```python
from build123d import *

# Parameters (mm, degrees)
CYLINDER001_R     = 1.5
CYLINDER001_DEPTH = 14
CYLINDER_R        = 1.5
CYLINDER_DEPTH    = 14
BOX003_W          = 3
BOX003_H          = 6.8
BOX003_DEPTH      = 6
BOX002_W          = 3
BOX002_H          = 6.8
BOX002_DEPTH      = 6
BOX001_W          = 3
BOX001_H          = 65
BOX001_DEPTH      = 6


with BuildPart() as cylinder001:
    # Cylinder001 → Cylinder001 (new body)
    with BuildSketch(Plane(origin=(-13, 30.6, 0), x_dir=(0, 0, -1), z_dir=(1, 0, 0))):
        Circle(CYLINDER001_R)
    extrude(amount=CYLINDER001_DEPTH)


with BuildPart() as cylinder:
    # Cylinder → Cylinder (new body)
    with BuildSketch(Plane(origin=(-13, -27.6, 0), x_dir=(0, 0, -1), z_dir=(1, 0, 0))):
        Circle(CYLINDER_R)
    extrude(amount=CYLINDER_DEPTH)


with BuildPart() as cube003:
    # Box003 → Box003 (new body)
    with BuildSketch(Plane(origin=(-6, -31, -3), x_dir=(1, 0, 0), z_dir=(0, 0, 1))):
        with Locations((1.5, 3.4)):
            Rectangle(BOX003_W, BOX003_H)
    extrude(amount=BOX003_DEPTH)


with BuildPart() as cube002:
    # Box002 → Box002 (new body)
    with BuildSketch(Plane(origin=(-6, 27.2, -3), x_dir=(1, 0, 0), z_dir=(0, 0, 1))):
        with Locations((1.5, 3.4)):
            Rectangle(BOX002_W, BOX002_H)
    extrude(amount=BOX002_DEPTH)


with BuildPart() as cut002:
    # Box001 → Box001 (new body)
    with BuildSketch(Plane(origin=(-3, -31, -3), x_dir=(1, 0, 0), z_dir=(0, 0, 1))):
        with Locations((1.5, 32.5)):
            Rectangle(BOX001_W, BOX001_H)
    extrude(amount=BOX001_DEPTH)

    # Fusion: union Cube003, Cube002
    add(cube003.part)
    add(cube002.part)

    # Cut001: cut Cylinder
    add(cylinder.part, mode=Mode.SUBTRACT)

    # Cut002: cut Cylinder001
    add(cylinder001.part, mode=Mode.SUBTRACT)


solid = cut002.part
```
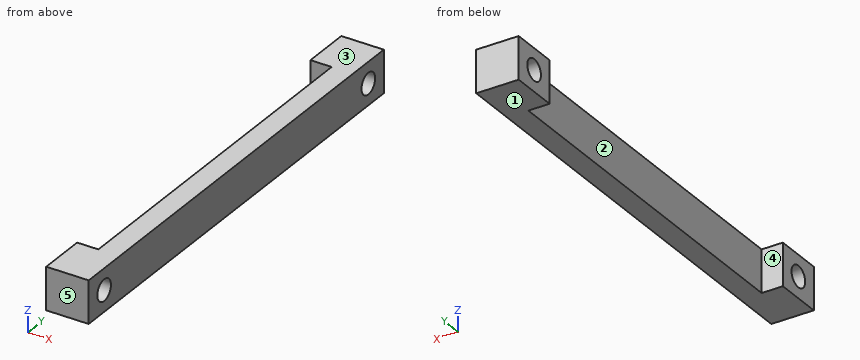
Geometry check sheet. Reference: the model listing, model coordinates, mm. Face numbers are marked on the shaded views. A direction names the side the tool comes from. Coordinates: 2 decimals unless noted, no trailing zeros. Order: outer loops, then holes, each group sorted by start corner. A loop starts at its lowest first (then second) coordinate and runs counter-clockwise, first axis right, second up. Notation, with made-up numbers: (65, 33.25) - (96, 33.25) arc R11 cw to (96, 54.25) - close; hole circle Ø11 at (-6, 3.5). An arc over 180 degrees is marked (long way). Answer in a Markdown table with one row per item. Add a question column.
1. Section check B-B (z = 0). Enter the section's corners in (x, y).
2. Section check C-C (y = -27.6). Enter the section's corners in (x, z), plus the area to 3 significant figures.
3. Section check A-A (x = -4.45). Enter the section's corners in (y, z).
4. Access from +Z, -Z, +X, -X, +Y, -Y to the whole of each face (thin tool, end or side, straight path). Record for the marked faces 1 and 2.
5. Material ranges on L1, parallel to Y at x = -2.5, z = 0; L2, parallel to Y at x = -3.8, z = 0; L3, parallel to Z at x = -2.95, y = 30.6, recorded low to high. Write a range as [from, to].
6. Gauge pin test, flat ends, axial feed: pin 1 Ø3 at (x, y) = (-4, -24) entering from -Z; pin 2 Ø1.8 at (y, z) = (30.6, 0) entering from -X. Record the tip position at first contact, or that the pin passes through.
7. Draft check along Y on the marked faces 3, 4 and 5. Enter one of: +Y half, -Y half, draft (parallel to the pull), parting line (faces both ways), or undercut.
8. Section check D-D (x = -1.65). Enter the section's corners in (y, z).
Data:
| question | item | result |
|---|---|---|
| 1 | outline | (-6, -31) - (0, -31) - (0, -29.1) - (-6, -29.1) - close; (-6, -26.1) - (0, -26.1) - (0, 29.1) - (-6, 29.1) - (-6, 27.2) - (-3, 27.2) - (-3, -24.2) - (-6, -24.2) - close; (-6, 32.1) - (0, 32.1) - (0, 34) - (-6, 34) - close |
| 2 | outline | (-6, -3) - (0, -3) - (0, -1.5) - (-6, -1.5) - close; (-6, 1.5) - (0, 1.5) - (0, 3) - (-6, 3) - close |
| 2 | area | 18.0 mm² |
| 3 | outline | (-31, -3) - (-24.2, -3) - (-24.2, 3) - (-31, 3) - close; (27.2, -3) - (34, -3) - (34, 3) - (27.2, 3) - close; hole circle Ø3 at (-27.6, 0); hole circle Ø3 at (30.6, 0) |
| 4 | face 1 | -Z, +X, -X, +Y, -Y |
| 4 | face 2 | +Z, -Z, -X |
| 5 | L1 | y = [-31, -29.1], [-26.1, 29.1], [32.1, 34] |
| 5 | L2 | y = [-31, -29.1], [-26.1, -24.2], [27.2, 29.1], [32.1, 34] |
| 5 | L3 | z = [-3, -1.5], [1.5, 3] |
| 6 | pin 1 | stops at z = -3 |
| 6 | pin 2 | passes through |
| 7 | face 3 | draft |
| 7 | face 4 | undercut |
| 7 | face 5 | -Y half |
| 8 | outline | (-31, -3) - (34, -3) - (34, 3) - (-31, 3) - close; hole circle Ø3 at (-27.6, 0); hole circle Ø3 at (30.6, 0) |
